Source: CAD feature listing. Evaluate the final solid. Frame: model axes, mm. A direction names the side the tool comes from. Give positions to 0.01 mm unless a question says otherwise; leave off trailing zeros. Order: outer loops, then holes, each group sorted by start corner. A loop starts at its lowest first (then second) coordinate and runs counter-clockwise, first axis right, second up. Notation, with made-up numbers: M 72.25,22 L 102.25,22 A20 ccw 102.25,34 Z; hole C 15.25,-10.5 d3. An arc over 180 degrees is marked long. Use CSV: the item, a comma, the result in double quotes. Start each with the question number.
Item 1: First-contact query: pin 1 (1 mm diameter, centred on x = -1, z = 0, fed in from -Y). Flat tip, straight axial feed; report the tip coordinate or a pass-through.
Item 2: Section query D-D on z = 3.5. Return loops of the section in (x, y), and give its area (3 significant figures).
Item 3: Pull-direction query (Z, two-part tool) for faces 3 (the face through (0.37, 0.74, 1.66)), 4 (the face through (0, 0, 2)), 5 (the face through (0, 1, -7.5)); classes: +Z half, -Z half, draft (parallel to the pull), parting line (faces both ways), or undercut.
Item 4: Section query B-B on x = 0. Return loops of the section in (y, z), and give its area (3 significant figures).
Item 5: Access query for faces 1 (the face through (0, 1.6, 2)), 2 (the face through (0.37, 0.74, 6.66)). Directions: +Z, -Z, +X, -X, +Y, -Y. A direction counts if a zero-diameter tool reaches every point of the face in a straight line with its end or side. Return the directions, or none.
Item 6: Section query C-C on z = 5. Return loops of the section in (x, y).
Item 7: Section query A-A on y = 0.9. Return loops of the section in (x, z), and give its area (3 significant figures).
Item 8: Ray query, probe 1 along Z at (x, y) = (0, 0.85); probe 2 along Z at (x, y) = (1.1, 1); probe 3 along X at (y, z) = (0.25, -4). Return the intervals inside material, ascending. Write a range as from..to.
Autodesk Inventor part; units mm, degrees
ref_plane "YZ Plane" through (0, 0, 0) normal (1, 0, 0) x (0, 1, 0)
ref_plane "XZ Plane" through (0, 0, 0) normal (0, 1, 0) x (-1, 0, 0)
ref_plane "XY Plane" through (0, 0, 0) normal (0, 0, 1) x (1, 0, 0)
sketch "草圖1" plane through (0, 0, 0) normal (0, 1, 0) x (-1, 0, 0)
  line L0 (2.5, 7.5) -> (-2.5, 7.5)
  line L1 (-2.5, 7.5) -> (-2.5, -7.5)
  line L2 (-2.5, -7.5) -> (2.5, -7.5)
  line L3 (2.5, -7.5) -> (2.5, 7.5)
  circle A0 centre (0, 5) radius 1.7
  line L4 (2.5, 0) -> (-2.5, 0) construction
  circle A1 centre (0, -5) radius 1.7
  circle A2 centre (0, 0) radius 1.7
  point P0 (0, 7.5)
  dimension "d0" = 5
  dimension "d1" = 15
  dimension "d2" = 3.4
  dimension "d3" = 2.5
  dimension "d4" = 2.5
  dimension "d9" = 3.4
extrude "擠出1" add sketch "草圖1" along normal blind 1.6 contours L3 L2 L1 L0 | A0 | A1 | A2
extrude "擠出2" cut sketch "草圖1" along normal blind 1.5 contours A0 | A1
extrude "擠出3" cut sketch "草圖1" along normal blind 1.5 contours A2
properties part number "110033226_ipt_08_平滑面(2x1)"
Verdict:
1,pin 1,"y = 1.5"
2,outline,"M -2.5,0 L -0.8,0 L -0.8,1.5 L 0.8,1.5 L 0.8,0 L 2.5,0 L 2.5,1.6 L -2.5,1.6 Z"
2,area,"5.60 mm2"
3,face 3,"undercut"
3,face 4,"draft"
3,face 5,"-Z half"
4,outline,"M 0,-7.5 L 1.6,-7.5 L 1.6,7.5 L 0,7.5 L 0,6.7 L 1.5,6.7 L 1.5,3.3 L 0,3.3 L 0,1.7 L 1.5,1.7 L 1.5,-1.7 L 0,-1.7 L 0,-3.3 L 1.5,-3.3 L 1.5,-6.7 L 0,-6.7 Z"
4,area,"8.70 mm2"
5,face 1,"+Z, -Z, +X, -X, +Y"
5,face 2,"-Y"
6,outline,"M -2.5,0 L -1.7,0 L -1.7,1.5 L 1.7,1.5 L 1.7,0 L 2.5,0 L 2.5,1.6 L -2.5,1.6 Z"
7,outline,"M -2.5,-7.5 L 2.5,-7.5 L 2.5,7.5 L -2.5,7.5 Z; hole C 0,-5 d3.4; hole C 0,0 d3.4; hole C 0,5 d3.4"
7,area,"47.8 mm2"
8,probe 1,"-7.5..-6.7, -3.3..-1.7, 1.7..3.3, 6.7..7.5"
8,probe 2,"-7.5..-6.3, -3.7..-1.3, 1.3..3.7, 6.3..7.5"
8,probe 3,"-2.5..-1.37, 1.37..2.5"
